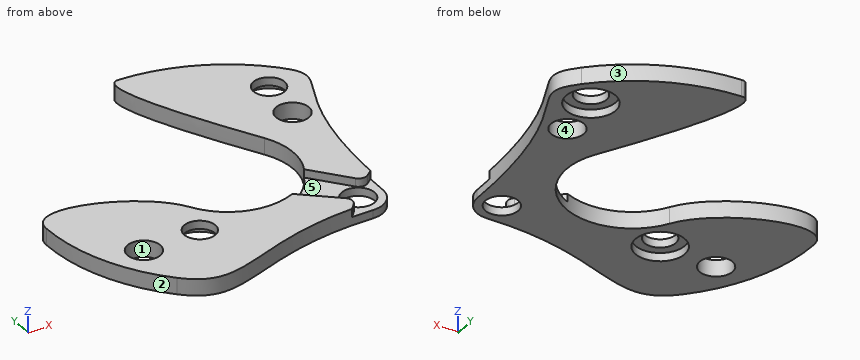
```python
from build123d import *

# Parameters (mm, degrees)
CROQUIS1_R                   = 0.5
SALIENTE_EXTRUIR1_DEPTH      = 0.5
CROQUIS3_R                   = 0.75
CORTAR_EXTRUIR1_DEPTH        = 0.25
CORTAR_EXTRUIR2_DEPTH        = 0.25
TALADRO_ROSCADO_M1_2X0_251_D = 0.95


with BuildPart() as part:
    # Croquis1 → Saliente-Extruir1 (new body)
    with BuildSketch(Plane.XY):
        with BuildLine():
            add(Edge.make_bspline(
                [(3.889087297, 3.889087297), (5.132893433, 2.64528116), (3.224873734, 3.014627212), (3.224873734, -2.474873734)],
                knots=[0, 0, 0, 0, 0.763896924, 0.763896924, 0.763896924, 0.763896924], degree=3))
            ThreePointArc((3.889087297, 3.889087297), (2.104758878, 5.081337429), (0, 5.5))
            add(Edge.make_bspline(
                [(1.732050808, 1), (0.948721344, 2.35676643), (-0.820788378, 5.5), (0, 5.5)],
                knots=[0, 0, 0, 0, 1, 1, 1, 1], degree=3))
            ThreePointArc((1.732050808, 1), (1, -1.732050808), (-1.732050808, -1))
            add(Edge.make_bspline(
                [(-1.732050808, -1), (-2.515380271, 0.35676643), (-5.5, 1.262116296), (-5.5, 0)],
                knots=[0, 0, 0, 0, 1, 1, 1, 1], degree=3))
            ThreePointArc((-5.5, 0), (-5.081337429, -2.104758878), (-3.889087297, -3.889087297))
            add(Edge.make_bspline(
                [(2.474873734, -3.224873734), (-1.35865781, -3.224873734), (-2.388951019, -5.389223574), (-3.889087297, -3.889087297)],
                knots=[0, 0, 0, 0, 1, 1, 1, 1], degree=3))
            ThreePointArc((2.474873734, -3.224873734), (3.00520382, -3.00520382), (3.224873734, -2.474873734))
        make_face()
        with Locations((-3.897114317, -2.25)):
            Circle(CROQUIS1_R, mode=Mode.SUBTRACT)
        with Locations((2.474873734, -2.474873734)):
            Circle(CROQUIS1_R, mode=Mode.SUBTRACT)
        with Locations((3.031088913, 1.75)):
            Circle(CROQUIS1_R, mode=Mode.SUBTRACT)
    extrude(amount=SALIENTE_EXTRUIR1_DEPTH)

    # Croquis3 → Cortar-Extruir1 (cut)
    with BuildSketch(Plane(origin=(0, 0, 0), x_dir=(-1, 0, 0), z_dir=(0, 0, -1))):
        with Locations((-3.181980515, 3.181980515)):
            Circle(CROQUIS3_R)
        with Locations((2.121320344, -2.121320344)):
            Circle(CROQUIS3_R)
    extrude(amount=-CORTAR_EXTRUIR1_DEPTH, mode=Mode.SUBTRACT)

    # Croquis4 → Cortar-Extruir2 (cut)
    with BuildSketch(Plane.XY.offset(0.5)):
        with BuildLine():
            Line((2.697199053, -1.961968819), (1.793528827, -0.88501658))
            ThreePointArc((1.793528827, -0.88501658), (1.414213562, -1.414213562), (0.88501658, -1.793528827))
            Line((0.88501658, -1.793528827), (1.961968819, -2.697199053))
            ThreePointArc((1.961968819, -2.697199053), (2.050320591, -2.866921228), (1.992783027, -3.049407066))
            Line((1.992783027, -3.049407066), (1.827745002, -3.246091726))
            add(Edge.make_bspline(
                [(2.474873734, -3.224873734), (2.249714916, -3.224873734), (2.034226396, -3.232340066), (1.827745002, -3.246091726)],
                knots=[0, 0, 0, 0, 0.058734046, 0.058734046, 0.058734046, 0.058734046], degree=3))
            ThreePointArc((2.474873734, -3.224873734), (3.00520382, -3.00520382), (3.224873734, -2.474873734))
            add(Edge.make_bspline(
                [(3.233875287, -1.837995811), (3.227985327, -2.041061917), (3.224873734, -2.253190531), (3.224873734, -2.474873734)],
                knots=[0.733048379, 0.733048379, 0.733048379, 0.733048379, 0.763896924, 0.763896924, 0.763896924, 0.763896924], degree=3))
            Line((3.233875287, -1.837995811), (3.049407066, -1.992783027))
            ThreePointArc((3.049407066, -1.992783027), (2.866921228, -2.050320591), (2.697199053, -1.961968819))
        make_face()
    extrude(amount=-CORTAR_EXTRUIR2_DEPTH, mode=Mode.SUBTRACT)

    # Taladro roscado M1.2x0.251 (through all)
    with Locations(Plane(origin=(0, 0, 0.25), x_dir=(-1, 0, 0), z_dir=(0, 0, -1))):
        with Locations((2.121320344, -2.121320344), (-3.181980515, 3.181980515)):
            Hole(TALADRO_ROSCADO_M1_2X0_251_D / 2)


solid = part.part
```
The listing builds one solid part. Answer for the finished solid, in the listing's coordinates (mm). Face numbers are marked on the shaded views. A direction names the side the tool comes from. Coordinates: 2 decimals unless noted, no trailing zeros. Answer as a JSON object with one key per item and string values. Group by question number.
Item 1: Each of these flat-tipped pins is pushed along its axis until it touches: P1, Ø1.2, axis at x = 3.18, y = 3.18, coming from the -Z side; P2, Ø5, axis at x = -3.5, y = 3.5, coming from the +Z side. Where does it stop, or does it pass through?
Item 2: Which of the six approach directions +Z, -Z, +X, -X, +Y, -Y give full straight-line access (tool end or side, diameter ignored) to the marked faces 4 and 5?
Item 3: Section A-A (y = -2.25) is taken. Give the number of separate pieces and of enclosed holes in the cut face, and give its area (3 significant figures).
Item 4: Determine the mould class of the marked faces 1, 2 and 3 for opening direction Y: +Y half, -Y half, draft (parallel to the pull), parting line (faces both ways), or undercut.
Item 5: Consider L1, parallel to Y at x = 0.75, z = 0.3; L2, parallel to Y at x = -3.5, z = 0.15; L3, parallel to X at y = -0.5, z = 0.35. Determine where each line is inside the solid, lowest interval first.
Solved:
{
 "1": {"P1": "stops at z = 0.25", "P2": "passes through"},
 "2": {"face 4": "+Z, -Z", "face 5": "+Z"},
 "3": {"separate pieces": "4", "enclosed holes": "0", "area": "2.35 mm2"},
 "4": {"face 1": "undercut", "face 2": "-Y half", "face 3": "+Y half"},
 "5": {"L1": "y = -3.38 to -1.85, 2.77 to 5.45", "L2": "y = -4.21 to -2.55, -1.95 to 0.34", "L3": "x = -5.48 to -2.14, 1.94 to 3.32"}
}
